Could you check a few things on this model? Use its own coordinates, in mm. Face numbers are marked on the shaded views. A direction names the side the tool comes from. Give positions to 0.01 mm unless a question says otherwise; leave off trailing zeros. Order: outer loops, then holes, each group sorted by start corner. A loop starts at its lowest first (then second) coordinate and runs counter-clockwise, first axis right, second up. Notation, with made-up numbers: M 41,-27.75 L 91,-27.75 A11 ccw 91,-22.75 Z; hole C -9.75,33 d4. An arc over 180 degrees is marked long. Use a Markdown table: item, result. Add a question column.
Item 1: If we mould it in two halves opening along Y, with no side actions, what happens to the marked faces 1, 2 and 3? For each: released by +Y, released by -Y, zero draft, split by the parting line, or undercut.
Item 2: Suppose I cut it at A-A on z = -27.5. Write out the boundary of the cut face in (x, y).
Item 3: For the marked faces 4 and 5, which set-ups out of +Z, -Z, +X, -X, +Y, -Y let a thin tool reach every point of the face, with its end or its side?
Item 4: Suppose I cut it at D-D on y = 16. Write out the boundary of the cut face in (x, z) (3 decimals), plus the area to 3 significant figures.
Item 5: Suppose I cut it at B-B on x = 15.5. Write out the boundary of the cut face in (y, z).
Item 6: If I drill on L1, parallel to Y at x = -5.5, z = -25; L2, parallel to Z at x = -13.25, y = -18.85 (3 decimals); L3, parallel to X at y = 18.5, z = -0.5 (3 decimals), over which ranges is the centre line in solid material (lowest first)? Write a range as from..to.
Item 7: I'm going to push flat-ended pins straight in: pin 1 Ø1.8 at (x, y) = (-12.5, 19) entering from +Z; pin 2 Ø14 at (x, y) = (-2.5, -8) entering from -Z; pin 3 Ø11 at (y, z) = (-10, -5) entering from +X (3 decimals). Where does each tip first touch, or does it pass through?
Item 8: Suppose I cut it at C-C on x = 3. Write out the boundary of the cut face in (y, z).
from build123d import *

# Parameters (mm, degrees)
F0_W      = 12.75
F0_H      = 40.5
F2_DEPTH  = 2
F3_START  = 18
F1_W      = 12.75
F1_H      = 20.25
F3_DEPTH  = 2.25
F4_START  = -18
F4_DEPTH  = 2.25
F6_DEPTH  = 2.25
F8_DEPTH  = 2.25
F9_R      = 1.125
F10_DEPTH = 40.501


with BuildPart() as f2:
    # F0 (on Top) → F2 (new body)
    with BuildSketch(Plane.XY):
        Rectangle(F0_W, F0_H)
    extrude(amount=F2_DEPTH)

    # F1 (on Front) → F3 (join)
    with BuildSketch(Plane.XZ.offset(F3_START)):
        with Locations((0, -10.125)):
            Rectangle(F1_W, F1_H)
    extrude(amount=F3_DEPTH)

    # F1 (on Front) → F4 (join)
    with BuildSketch(Plane.XZ.offset(F4_START)):
        with Locations((0, -10.125)):
            Rectangle(F1_W, F1_H)
    extrude(amount=-F4_DEPTH)

    # F5 (on face) → F6 (join, through all)
    with BuildSketch(Plane(origin=(0, 20.25, 0), x_dir=(-1, 0, 0), z_dir=(0, 1, 0))):
        Polygon((-6.375, -20.25), (-20.25, -20.25), (-20.25, -30.25), (20.25, -30.25), (20.25, -20.25), (6.375, -20.25), align=None)
    extrude(amount=-F6_DEPTH)

    # F7 (on face) → F8 (join, through all)
    with BuildSketch(Plane.XZ.offset(20.25)):
        Polygon((0, -20.25), (-20.25, -20.25), (-20.25, -30.25), (20.25, -30.25), (20.25, -20.25), align=None)
    extrude(amount=-F8_DEPTH)

    # F9 (on face) → F10 (cut, through all)
    with BuildSketch(Plane.XZ.offset(20.25)):
        with Locations((-13.25, -25.25)):
            Circle(F9_R)
        with Locations((13.25, -25.25)):
            Circle(F9_R)
    extrude(amount=-F10_DEPTH, mode=Mode.SUBTRACT)


solid = f2.part
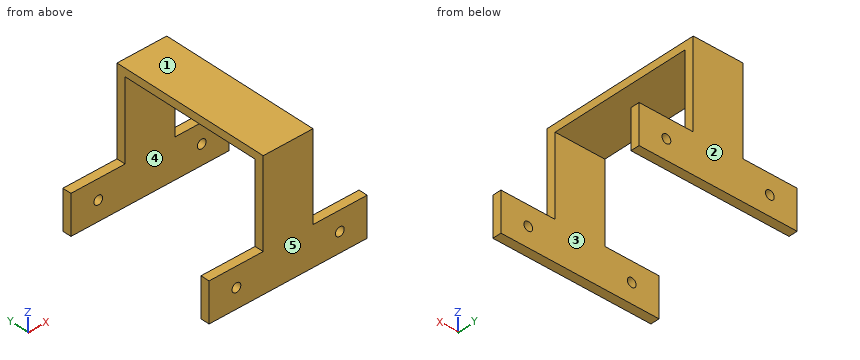
Findings below:
| question | item | result |
|---|---|---|
| 1 | face 1 | zero draft |
| 1 | face 2 | released by +Y |
| 1 | face 3 | undercut |
| 2 | outline | M -20.25,-20.25 L 20.25,-20.25 L 20.25,-18 L -20.25,-18 Z; M -20.25,18 L 20.25,18 L 20.25,20.25 L -20.25,20.25 Z |
| 3 | face 4 | -Z, +X, -X |
| 3 | face 5 | +Z, -Z, +X, -X, -Y |
| 4 | outline | M -6.375,0 L 6.375,0 L 6.375,2 L -6.375,2 Z |
| 4 | area | 25.5 mm^2 |
| 5 | outline | M -20.25,-30.25 L -18,-30.25 L -18,-20.25 L -20.25,-20.25 Z; M 18,-30.25 L 20.25,-30.25 L 20.25,-20.25 L 18,-20.25 Z |
| 6 | L1 | y = -20.25..-18, 18..20.25 |
| 6 | L2 | z = -30.25..-26.375, -24.125..-20.25 |
| 6 | L3 | x = -6.375..6.375 |
| 7 | pin 1 | stops at z = -20.25 |
| 7 | pin 2 | stops at z = 0 |
| 7 | pin 3 | stops at x = 6.375 |
| 8 | outline | M -20.25,-30.25 L -18,-30.25 L -18,0 L 18,0 L 18,-30.25 L 20.25,-30.25 L 20.25,2 L -20.25,2 Z |
